The listing builds one solid part. Answer for the finished solid, in the listing's coordinates (mm). A direction names the side the tool comes from. Give positions to 0.01 mm unless a question says otherwise; leave off trailing zeros. Write each loop counter-clockwise with the first axis right and the second up, starting at its lowest first coordinate (ties: lowest second). Pieces come first, ordered by that corner, then holes. Notation, with made-up numbers: (12, 58.5) -> (46, 58.5) arc R37 cw to (46, 97.5) -> close; hole circle Ø11 at (77.25, 8.5). An arc over 180 degrees is marked (long way). Put each result on its own line as item: value. Start each with the question number.
1) A cutting plane is placed at C-C (z = -12). Write down the section's boundary in (x, y), then the cut area to 3 significant figures.
2) Find the intervals of material crossed by line 1 along Y through (x, z) = (15.5, 3.1); line 2 along Y through (x, z) = (15.5, 1); line 3 along Y through (x, z) = (-1.5, -3.5), in increasing order. Write a range as from..to.
3) For faces 4 (the flat face through (0, 12, 0)), 5 (the flat face through (0, -23.5, -14)), determine the directions among +Z, -Z, +X, -X, +Y, -Y from which every point of the face is accessible in a straight line to the end or side of a thin tool.
4) A flat-ended cylindrical pin translates along its axis: pin 1 Ø4 at (x, y) = (-15.5, -15.5) entering from -Z. Find the tip coordinate at first contact, or state that the pin passes through.
5) For a pull along X with two mould halves and no side action, classify faces 1 (the flat face through (-21, -11, 3)), 2 (the cylindrical face through (-13.93, -20.96, -16.5)), 3 (the flat face through (0, -21, -30)) as released by +X, released by -X, zero draft, split by the parting line, or undercut.
6) A cutting plane is placed at B-B (y = -15.5). Write down the section's boundary in (x, z).
7) A cutting plane is placed at D-D (y = 20). Write down the section's boundary in (x, z).
8) A cutting plane is placed at A-A (x = 0). Write down the section's boundary in (y, z).
from build123d import *

# Parameters (mm, degrees)
ESQUISSE1_R             = 10.5
BOSS_EXTRU_1_DEPTH      = 5
ESQUISSE2_W             = 42
ESQUISSE2_H             = 5
BOSS_EXTRU_2_DEPTH      = 30
ESQUISSE3_R             = 1.5
ENL_V_MAT_EXTRU_1_DEPTH = 30
CONG_1_R                = 10
CONG_2_R                = 3
ESQUISSE4_R             = 1.5
ESQUISSE4_R_2           = 1.499999579
ENL_V_MAT_EXTRU_2_DEPTH = 44.511492735
CONG_3_R                = 1.5


with BuildPart() as part:
    # Esquisse1 → Boss.-Extru.1 (new body)
    with BuildSketch(Plane.XY):
        with BuildLine():
            Line((-13, 23.5), (13, 23.5))
            ThreePointArc((13, 23.5), (18.656854249, 21.156854249), (21, 15.5))
            Line((21, 15.5), (21, -23.5))
            Line((21, -23.5), (-21, -23.5))
            Line((-21, -23.5), (-21, 15.5))
            ThreePointArc((-21, 15.5), (-18.656854249, 21.156854249), (-13, 23.5))
        make_face()
        Circle(ESQUISSE1_R, mode=Mode.SUBTRACT)
    extrude(amount=BOSS_EXTRU_1_DEPTH)

    # Esquisse2 → Boss.-Extru.2 (add)
    with BuildSketch(Plane(origin=(0, 0, 0), x_dir=(-1, 0, 0), z_dir=(0, 0, -1))):
        with Locations((0, -21)):
            Rectangle(ESQUISSE2_W, ESQUISSE2_H)
    extrude(amount=BOSS_EXTRU_2_DEPTH)

    # Esquisse3 → Enlèv. mat.-Extru.1 (cut)
    with BuildSketch(Plane(origin=(0, -18.5, 0), x_dir=(1, 0, 0), z_dir=(0, 1, 0))):
        with Locations(Location((-14, 15, 0), (0, 0, 270))):
            Circle(ESQUISSE3_R)
        with Locations(Location((14, 15, 0), (0, 0, 270))):
            Circle(ESQUISSE3_R)
    extrude(amount=-ENL_V_MAT_EXTRU_1_DEPTH, mode=Mode.SUBTRACT)

    # Congé1
    cong_1_edges = [part.edges().sort_by_distance(p)[0] for p in [
        (-21, -21, -30),
        (21, -21, -30),
    ]]
    fillet(cong_1_edges, radius=CONG_1_R)

    # Congé2
    cong_2_edges = [part.edges().sort_by_distance(p)[0] for p in [
        (0, -23.5, 5),
    ]]
    fillet(cong_2_edges, radius=CONG_2_R)

    # Esquisse4 → Enlèv. mat.-Extru.2 (cut, through all)
    with BuildSketch(Plane(origin=(0, 0, 0), x_dir=(-1, 0, 0), z_dir=(0, 0, -1))):
        with Locations((-15.5, 15.5)):
            Circle(ESQUISSE4_R)
        with Locations((15.5, 15.5)):
            Circle(ESQUISSE4_R)
        with Locations((-15.499999687, -15.500000313)):
            Circle(ESQUISSE4_R_2)
        with Locations((15.5, -15.5)):
            Circle(ESQUISSE4_R)
    extrude(amount=-ENL_V_MAT_EXTRU_2_DEPTH, mode=Mode.SUBTRACT)

    # Congé3
    cong_3_edges = [part.edges().sort_by_distance(p)[0] for p in [
        (-10.5, 0, 5),
    ]]
    fillet(cong_3_edges, radius=CONG_3_R)


solid = part.part
Reply:
1. outline: (-21, -23.5) -> (21, -23.5) -> (21, -18.5) -> (-21, -18.5) -> close
1. area: 210 mm2
2. line 1: y = -23.29..-17, -14..14, 17..23.1
2. line 2: y = -23.5..-17, -14..14, 17..23.1
2. line 3: y = -23.5..-18.5
3. face 4: -Z, +X, -X, +Y
3. face 5: +Z, -Z, +X, -X, -Y
4. pin 1: stops at z = 0
5. face 1: released by -X
5. face 2: undercut
5. face 3: zero draft
6. outline: (-21, 0) -> (-17, 0) -> (-17, 5) -> (-21, 5) -> close; (-14, 0) -> (14, 0) -> (14, 5) -> (-14, 5) -> close; (17, 0) -> (21, 0) -> (21, 5) -> (17, 5) -> close
7. outline: (-19.61, 0) -> (19.61, 0) -> (19.61, 5) -> (-19.61, 5) -> close
8. outline: (-23.5, -30) -> (-18.5, -30) -> (-18.5, 0) -> (-10.5, 0) -> (-10.5, 3.5) arc R1.5 ccw to (-12, 5) -> (-20.5, 5) arc R3 ccw to (-23.5, 2) -> close; (10.5, 0) -> (23.5, 0) -> (23.5, 5) -> (12, 5) arc R1.5 ccw to (10.5, 3.5) -> close
